from build123d import *

# Parameters (mm, degrees)
SKIZZE2_R                       = 25
AUFSATZ_LINEAR_AUSTRAGEN2_DEPTH = 3
AUFSATZ_LINEAR_AUSTRAGEN1_DEPTH = 5


with BuildPart() as part:
    # Skizze2 → Aufsatz-Linear austragen2 (new body)
    with BuildSketch(Plane(origin=(0, 0, 0), x_dir=(1, 0, 0), z_dir=(0, 1, 0))):
        Circle(SKIZZE2_R)
    extrude(amount=AUFSATZ_LINEAR_AUSTRAGEN2_DEPTH)

    # Model → Aufsatz-Linear austragen1 (add)
    with BuildSketch(Plane(origin=(0, 3, -3), x_dir=(1, 0, 0), z_dir=(0, -1, 0))):
        Polygon((-4.104544089, 5.371303079), (-1.178372214, 1.279701516), (-15.653137839, -8.684400046), (-22.055559714, 2.361810891), (-11.094544089, 21.499584329), (10.959909036, 21.497357766), (13.499830911, 17.115131204), (9.924205911, 14.669310891), (8.470377786, 17.177592141), (-8.590481589, 17.179349954), (-17.069700339, 2.374701516), (-15.335325339, -0.617798484), (-7.115325339, 3.386615579), (-10.358840964, 8.025599954), (7.050534036, 12.703842141), align=None)
        Polygon((15.672018411, 13.367240579), (10.169830911, 9.603646829), (1.176393411, 3.438998391), (4.118971536, -0.680845359), (-5.261184714, -6.810220359), (-7.008684714, -8.005532859), (10.356862161, -3.306900046), (7.113346536, 1.332084329), (15.428268411, 5.173021829), (17.067721536, 2.344232766), (8.588502786, -12.460650046), (-8.472356589, -12.458657859), (-9.905090964, -9.986704734), (-13.480715964, -12.432525046), (-10.961887839, -16.778423484), (11.092565286, -16.780884421), (22.053346536, 2.357123391), align=None)
    extrude(amount=-AUFSATZ_LINEAR_AUSTRAGEN1_DEPTH)


solid = part.part
Build history of the part. All positions in model axes, mm. A direction names the side the tool comes from. Round coordinates to 2 decimals unless told otherwise and drop trailing zeros. Write each loop counter-clockwise with the first axis right and the second up, starting at its lowest first coordinate (ties: lowest second). Pieces come first, ordered by that corner, then holes. Notation, with made-up numbers: M 54.5,54.25 L 82.5,54.25 A17 ccw 82.5,76.25 Z; hole C 1,47.5 d2. An arc over 180 degrees is marked long. Answer as a JSON object with one key per item and string values. Group by question number.
(1) Cut at D-D (y = 1.75). Give the cut face in (x, z).
(2) Drill centre lines: L1, parallel to Z at x = -12, y = 6.75; L2, parallel to Z at x = 5, y = 3.5; L3, parallel to X at y = 6, z = 14. Where is each one in solid material? Low to high.
(3) Mould opens along Z. For faces 6 (the flat face through (2.627, 5.465, -1.592)), 7 (the flat face through (12.21, 5.46, 16.34)), 8 (the flat face through (16.496, 5.465, -10.346)) say: pulls with the +Z half, pulls with the -Z half, needs draft (parallel to the pull), parting line crosses it, or undercut.
(4) Which spindle directions (+Z, -Z, +X, -X, +Y, -Y) get a long thin tool onto all of the face, cutting with end or side? Do faces 1 (the flat face through (-2.66, 5.46, 0.35)), 2 (the flat face through (7, 8, -7)), 3 (the flat face through (18.9, 5.5, 4.8)), 4 (the flat face through (-18.81, 5.46, -6.24)), 5 (the flat face through (-11.668, 5.465, -14.192)). Say none if no direction does.
(5) Cut at B-B (z = -8). Give the cut face in (x, y).
(6) Flat gauge pins, fed straight in: pin 1 (1 mm diameter, centred on x = -11.5, y = 5, fed in from -Z); pin 2 (1.5 mm diameter, centred on x = 7, y = 5.5, fed in from -Z); pin 3 (3 mm diameter, centred on y = 2.5, z = -12, fed in from +X). Where does each tip first touch, or does it go through?
(7) Cut at C-C (x = 14.5). Give the cut face in (y, z).
Responses:
{
 "1": {"outline": "C 0,0 d50"},
 "2": {"L1": "z = -17.99 to -14.42, -9.17 to -1.99, 8.23 to 16.92", "L2": "z = -19.78 to -15.46, -7.76 to 3.06, 8.36 to 9.15, 14.18 to 18.5", "L3": "x = -13.67 to -8.69, 8.57 to 13.33"},
 "3": {"face 6": "undercut", "face 7": "pulls with the +Z half", "face 8": "pulls with the -Z half"},
 "4": {"face 1": "+Y", "face 2": "+Z, -Z, +X, -X, +Y", "face 3": "+Z, +X, +Y", "face 4": "-Z, -X, +Y", "face 5": "-X, +Y"},
 "5": {"outline": "M -23.69,0 L 23.69,0 L 23.69,3 L 17.84,3 L 17.84,8 L 12.86,8 L 12.86,3 L 4.1,3 L 4.1,8 L -2.49,8 L -2.49,3 L -10.3,3 L -10.3,8 L -17.79,8 L -17.79,3 L -23.69,3 Z"},
 "6": {"pin 1": "stops at z = -19.71", "pin 2": "stops at z = -19.78", "pin 3": "stops at x = 22.69"},
 "7": {"outline": "M 0,-20.37 L 3,-20.37 L 3,-13.83 L 8,-13.83 L 8,-5.14 L 3,-5.14 L 3,1.74 L 8,1.74 L 8,9.57 L 3,9.57 L 3,20.37 L 0,20.37 Z"}
}
